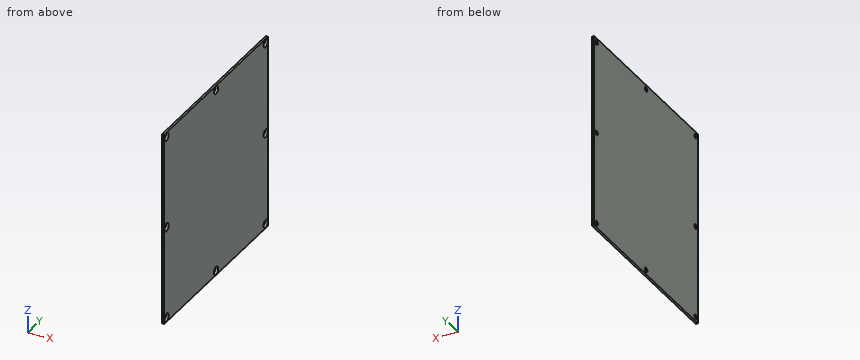
Autodesk Inventor part; units mm, degrees
ref_plane "YZ Plane" through (0, 0, 0) normal (1, 0, 0) x (0, 1, 0)
ref_plane "XZ Plane" through (0, 0, 0) normal (0, 1, 0) x (-1, 0, 0)
ref_plane "XY Plane" through (0, 0, 0) normal (0, 0, 1) x (1, 0, 0)
sketch "Sketch1" plane through (0, 0, 0) normal (1, 0, 0) x (0, 1, 0)
  line L0 (-69.85, -69.85) -> (69.85, -69.85)
  line L1 (69.85, -69.85) -> (69.85, 69.85)
  line L2 (69.85, 69.85) -> (-69.85, 69.85)
  line L3 (-69.85, 69.85) -> (-69.85, -69.85)
  line L4 (-69.85, -69.85) -> (69.85, 69.85) construction
  line L5 (69.85, -69.85) -> (-69.85, 69.85) construction
  point P0 (0, 0)
  dimension "d0" = 139.7
  dimension "d1" = 139.7
extrude "Extrusion1" add sketch "Sketch1" along normal blind 1.5875
sketch "Sketch6" plane through (1.5875, 0, 0) normal (1, 0, 0) x (0, 0, -1)
  line L0 (69.85, -69.85) -> (69.85, 69.85)
  line L1 (69.85, 69.85) -> (-69.85, 69.85)
  line L2 (-69.85, 69.85) -> (-69.85, -69.85)
  line L3 (-69.85, -69.85) -> (69.85, -69.85)
  point P0 (0, 0)
  point P1 (-66.675, -66.675)
  point P2 (-66.675, 0)
  dimension "d45" = 3.175
  dimension "d46" = 3.175
  dimension "d57" = 69.85
hole "Hole4" at (1.5875, -66.675, 66.675) at (1.5875, 0, 66.675) direction (-1, 0, 0) diameter 3.2766 end through all countersink diameter 5.715 countersink angle 82
pattern_circular "Circular Pattern1" count 4 over 360 about axis through (-10, 0, 0) along (1, 0, 0) of "Hole4"
equation "\"d0\" = width + 2 * plasticThickness"
equation "\"d1\" = height + 2 * plasticThickness"
equation "\"d2\" = frontPanelThickness"
equation "\"height\" = 127"
equation "\"width\" = 127"
equation "\"plasticThickness\" = 6.35"
equation "\"caseThickness\" = 6.35"
equation "\"alignmentGrooveDepth\" = 1.5875"
equation "\"alignmentGrooveClearance\" = 0.1016"
equation "\"aerogelHolderDepth\" = 49.022"
equation "\"depth\" = 203.2"
equation "\"mirrorAngle\" = 2.5deg"
equation "\"mirrorThickness\" = 3.175"
equation "\"fresnelThickness\" = 0.254"
equation "\"focalLength\" = 152.4"
equation "\"ior\" = 1.49"
equation "\"centerThickness\" = 1.27"
equation "\"fresnelAngle\" = 90deg"
equation "\"fresnelEffectiveDiameter\" = 152.4"
equation "\"frontPanelThickness\" = 1.5875"
equation "\"fresnelGrooveWidth\" = 1.778"
properties part number "front" material "Aluminum 6061"
Check sheet for the modelled part. Datum: model origin and axes. Units: mm. Round coordinates to 2 decimals unless told otherwise and drop trailing zeros. Order: outer loops, then holes, each group sorted by start corner. A loop starts at its lowest first (then second) coordinate and runs counter-clockwise, first axis right, second up. Notation, with made-up numbers: (0, -4) - (17, -4) arc R25 ccw to (17, 27) - close; hole circle Ø9 at (16, 49). An arc over 180 degrees is marked (long way). Write item = value, one per line.
Q1. Section check A-A (z = 0). Record the boundary of the cut face in (x, y), and give its area (3 significant figures).
Computed:
outline = (0, -69.85) - (1.59, -69.85) - (1.59, -69.53) - (0.18, -68.31) - (0, -68.31) - close; (0, -65.04) - (0.18, -65.04) - (1.59, -63.82) - (1.59, 63.82) - (0.18, 65.04) - (0, 65.04) - close; (0, 68.31) - (0.18, 68.31) - (1.59, 69.53) - (1.59, 69.85) - (0, 69.85) - close
area = 208 mm^2
Q2. Thickness scan on line 1 along Y through (x, z) = (0.2, -1). Record the ranges inside material, lowest first.
Computed:
line_1 = -69.85 to -67.99, -65.36 to 65.36, 67.99 to 69.85
Q3. Go/stop test with flat-tipped pins: pin 1 (5 mm diameter, centred on y = 66.675, z = -66.675, fed in from +X); pin 2 (1.5 mm diameter, centred on y = 22, z = -25, fed in from -X); pin 3 (2 mm diameter, centred on y = 0, z = -66.675, fed in from -X); pin 4 (4.5 mm diameter, centred on y = 0, z = 66.675, fed in from +X). Record where each tip stops, or that it passes through.
Computed:
pin_1 = 1.18
pin_2 = 0
pin_3 = through
pin_4 = 0.89
